Here's how the part is built. I have some questions about the finished solid (model axes, mm). Round coordinates to 2 decimals unless told otherwise and drop trailing zeros. Loops run counter-clockwise (first coordinate to the right, second up) from the corner with the lowest first, then second, coordinate; pieces in that order, holes last. Notation, with made-up numbers: (-7.5, 60.25) - (43.5, 60.25) arc R15 ccw to (43.5, 70.25) - close; hole circle Ø7 at (85, 54). An arc over 180 degrees is marked (long way). Return JSON: item names as keys, results as strings. Group by question number.
```python
from build123d import *

# Parameters (mm, degrees)
SKETCH1_W           = 67
SKETCH1_H           = 40
SKETCH1_R           = 1.2
SKETCH1_W_2         = 5
SKETCH1_H_2         = 20
SKETCH1_W_3         = 36.5
SKETCH1_R_2         = 1.197563381
SKETCH1_R_3         = 1.7
SKETCH1_R_4         = 5
BOSS_EXTRUDE2_DEPTH = 3


with BuildPart() as part:
    # Sketch1 → Boss-Extrude2 (new body)
    # profile 1 of 3: a face of its own
    with BuildSketch(Plane(origin=(0, 0, 0), x_dir=(1, 0, 0), z_dir=(0, 1, 0))):
        Rectangle(SKETCH1_W, SKETCH1_H)
        with Locations(Location((-30, -17.5, 0), (0, 0, 270))):
            Circle(SKETCH1_R, mode=Mode.SUBTRACT)
        with Locations(Location((-13.5, -17.5, 0), (0, 0, 270))):
            Circle(SKETCH1_R, mode=Mode.SUBTRACT)
        with Locations(Location((13.5, -17.5, 0), (0, 0, 270))):
            Circle(SKETCH1_R, mode=Mode.SUBTRACT)
        with Locations(Location((30, -17.5, 0), (0, 0, 270))):
            Circle(SKETCH1_R, mode=Mode.SUBTRACT)
        Rectangle(SKETCH1_W_2, SKETCH1_H_2, mode=Mode.SUBTRACT)
        with Locations(Location((-30, 17.5, 0), (0, 0, 270))):
            Circle(SKETCH1_R, mode=Mode.SUBTRACT)
        with Locations(Location((-13.5, 17.5, 0), (0, 0, 270))):
            Circle(SKETCH1_R, mode=Mode.SUBTRACT)
        with Locations(Location((13.5, 17.5, 0), (0, 0, 270))):
            Circle(SKETCH1_R, mode=Mode.SUBTRACT)
        with Locations(Location((30, 17.5, 0), (0, 0, 270))):
            Circle(SKETCH1_R, mode=Mode.SUBTRACT)
    # profile 2 of 3: a face of its own
    with BuildSketch(Plane(origin=(0, 0, 0), x_dir=(1, 0, 0), z_dir=(0, 1, 0))):
        with Locations((-51.75, 0)):
            Rectangle(SKETCH1_W_3, SKETCH1_H)
        with Locations(Location((-61.75, -17.5, 0), (0, 0, 270))):
            Circle(SKETCH1_R_2, mode=Mode.SUBTRACT)
        with Locations(Location((-45.25, -17.5, 0), (0, 0, 270))):
            Circle(SKETCH1_R_2, mode=Mode.SUBTRACT)
        with Locations(Location((-61.75, -9, 0), (0, 0, 270))):
            Circle(SKETCH1_R_3, mode=Mode.SUBTRACT)
        with Locations(Location((-45.25, -9, 0), (0, 0, 270))):
            Circle(SKETCH1_R_3, mode=Mode.SUBTRACT)
        with Locations(Location((-53.5, 0, 0), (0, 0, 270))):
            Circle(SKETCH1_R_4, mode=Mode.SUBTRACT)
        with Locations(Location((-61.75, 9, 0), (0, 0, 270))):
            Circle(SKETCH1_R_3, mode=Mode.SUBTRACT)
        with Locations(Location((-45.25, 9, 0), (0, 0, 270))):
            Circle(SKETCH1_R_3, mode=Mode.SUBTRACT)
        with Locations(Location((-61.75, 17.5, 0), (0, 0, 270))):
            Circle(SKETCH1_R_2, mode=Mode.SUBTRACT)
        with Locations(Location((-45.25, 17.5, 0), (0, 0, 270))):
            Circle(SKETCH1_R_2, mode=Mode.SUBTRACT)
    # profile 3 of 3: a face of its own
    with BuildSketch(Plane(origin=(0, 0, 0), x_dir=(1, 0, 0), z_dir=(0, 1, 0))):
        with Locations((51.75, 0)):
            Rectangle(SKETCH1_W_3, SKETCH1_H)
        with Locations(Location((45.25, -17.5, 0), (0, 0, 270))):
            Circle(SKETCH1_R_2, mode=Mode.SUBTRACT)
        with Locations(Location((61.75, -17.5, 0), (0, 0, 270))):
            Circle(SKETCH1_R_2, mode=Mode.SUBTRACT)
        with Locations(Location((45.25, -9, 0), (0, 0, 270))):
            Circle(SKETCH1_R_3, mode=Mode.SUBTRACT)
        with Locations(Location((61.75, -9, 0), (0, 0, 270))):
            Circle(SKETCH1_R_3, mode=Mode.SUBTRACT)
        with Locations(Location((53.5, 0, 0), (0, 0, 270))):
            Circle(SKETCH1_R_4, mode=Mode.SUBTRACT)
        with Locations(Location((45.25, 9, 0), (0, 0, 270))):
            Circle(SKETCH1_R_3, mode=Mode.SUBTRACT)
        with Locations(Location((61.75, 9, 0), (0, 0, 270))):
            Circle(SKETCH1_R_3, mode=Mode.SUBTRACT)
        with Locations(Location((45.25, 17.5, 0), (0, 0, 270))):
            Circle(SKETCH1_R_2, mode=Mode.SUBTRACT)
        with Locations(Location((61.75, 17.5, 0), (0, 0, 270))):
            Circle(SKETCH1_R_2, mode=Mode.SUBTRACT)
    extrude(amount=BOSS_EXTRUDE2_DEPTH)


solid = part.part
```
Q1. Please list where these lines run through material, in increasing order: line 1 (X direction, y = 2.25, z = 9); line 2 (X direction, y = 0.1, z = 6); line 3 (Z direction, x = -29, y = 1.1).
Q2. Will this pin go through, and if not, where does the flat tip stop? pin 1 Ø1.4 at (x, z) = (13.5, 17.5) entering from +Y.
Q3. Imagine slicing it at B-B, the plane y = 1.3. Give the number of separate pieces and of enclosed holes in the cut face, and give its area (3 significant figures).
Q4. Imagine slicing it at C-C, the plane z = 0. List the corners of the cut face in (x, y) for me, and give its area (3 significant figures).
Q5. Imagine slicing it at A-A, the plane x = 53.5. List the corners of the cut face in (y, z) for me, and give its area (3 significant figures).
Q6. If we mould it in two halves opening along Z, with no side actions, what happens to faces 1 (the cylindrical face through (-48.543, 1.479, -0.651)), 2 (the flat face through (-1, 1, -20)), 3 (the flat face through (70, 1, 0))? For each: +Z half, -Z half, draft (parallel to the pull), parting line (faces both ways), or undercut.
Q7. Imagine slicing it at D-D, the plane x = 13.5. List the corners of the cut face in (y, z) for me, and give its area (3 significant figures).
Output values:
{
 "1": {"line 1": "x = -70 to -63.45, -60.05 to -46.95, -43.55 to -2.5, 2.5 to 43.55, 46.95 to 60.05, 63.45 to 70", "line 2": "x = -70 to -2.5, 2.5 to 70", "line 3": "z = -20 to -18.16, -16.84 to 16.84, 18.16 to 20"},
 "2": {"pin 1": "passes through"},
 "3": {"separate pieces": "1", "enclosed holes": "27", "area": "5,200 mm^2"},
 "4": {"outline": "(-70, 0) - (-58.5, 0) - (-58.5, 3) - (-70, 3) - close; (-48.5, 0) - (-2.5, 0) - (-2.5, 3) - (-48.5, 3) - close; (2.5, 0) - (48.5, 0) - (48.5, 3) - (2.5, 3) - close; (58.5, 0) - (70, 0) - (70, 3) - (58.5, 3) - close", "area": "345 mm^2"},
 "5": {"outline": "(0, -20) - (3, -20) - (3, -5) - (0, -5) - close; (0, 5) - (3, 5) - (3, 20) - (0, 20) - close", "area": "90.0 mm^2"},
 "6": {"face 1": "undercut", "face 2": "-Z half", "face 3": "draft"},
 "7": {"outline": "(0, -20) - (3, -20) - (3, -18.7) - (0, -18.7) - close; (0, -16.3) - (3, -16.3) - (3, 16.3) - (0, 16.3) - close; (0, 18.7) - (3, 18.7) - (3, 20) - (0, 20) - close", "area": "106 mm^2"}
}
